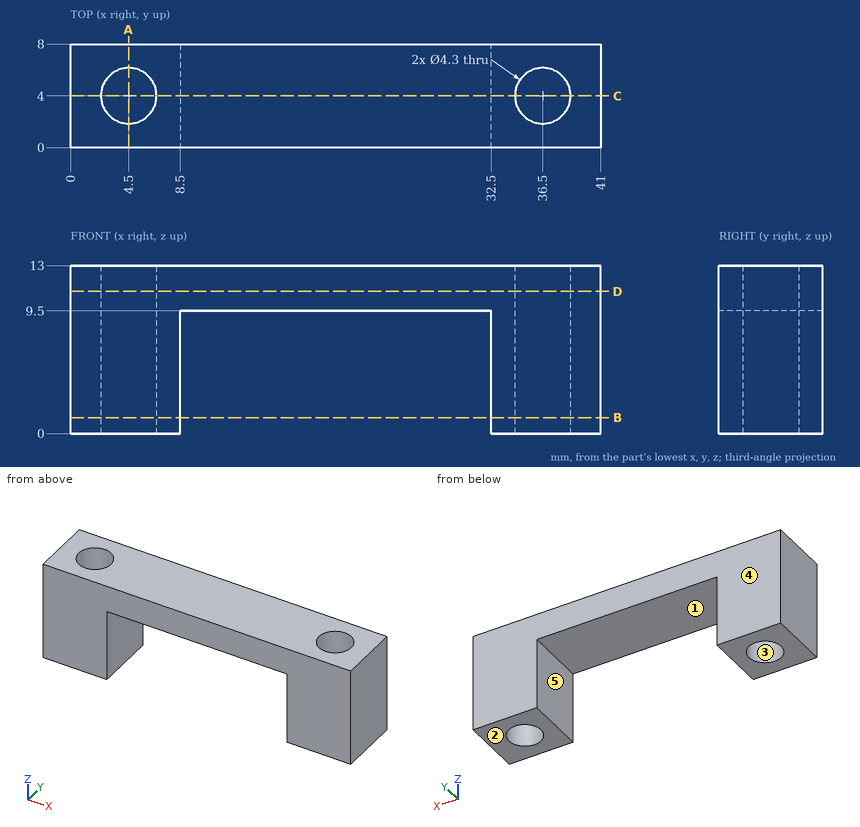
Drawing for the job (mm, zero at the part's lowest x, y, z). A direction names the side the tool comes from. Round coordinates to 2 decimals unless told otherwise and drop trailing zeros. Write each loop counter-clockwise with the first axis right and the second up, starting at its lowest first coordinate (ties: lowest second). Pieces come first, ordered by that corner, then holes. Notation, with made-up numbers: (4, -35.5) - (52, -35.5) arc R21 cw to (52, -1.5) - close; hole circle Ø11 at (24, 25). An arc over 180 degrees is marked (long way). Return JSON: item names as keys, results as strings. Group by question number.
Item 1: Band-saw the part on A-A on x = 4.5. List the corners of the cut face in (y, z), plus the area to 3 significant figures.
Item 2: Mould opens along Y. For the marked faces 3, 4 and 5 say: +Y half, -Y half, draft (parallel to the pull), parting line (faces both ways), or undercut.
Item 3: Flat gauge pins, fed straight in: pin 1 Ø1 at (x, y) = (26.5, 7) entering from -Z; pin 2 Ø2.5 at (x, y) = (36.5, 4) entering from +Z; pin 3 Ø2 at (y, z) = (5.5, 5.5) entering from -X. Where does each tip first touch, or does it go through?
Item 4: 3-axis set-ups, long thin cutter, end or side, ignore diameter. For the marked faces 1 and 2: which of +Z, -Z, +X, -X, +Y, -Y reach the whole face in a straight line?
Item 5: Band-saw the part on B-B on z = 1.25. List the corners of the cut face in (x, y).
Item 6: Band-saw the part on C-C on y = 4. List the corners of the cut face in (x, z).
Item 7: Probe probe 1 along Y at (x, z) = (4.5, 5.5); probe 2 along X at (y, z) = (1.75, 6.75); probe 3 along X at (y, z) = (4.5, 9.75). List the from-to ranges inside material, lowest first.
Item 8: Band-saw the part on D-D on z = 11. List the corners of the cut face in (x, y), plus the area to 3 significant figures.
Resolved:
{
 "1": {"outline": "(0, 0) - (1.85, 0) - (1.85, 13) - (0, 13) - close; (6.15, 0) - (8, 0) - (8, 13) - (6.15, 13) - close", "area": "48.1 mm²"},
 "2": {"face 3": "undercut", "face 4": "+Y half", "face 5": "draft"},
 "3": {"pin 1": "stops at z = 9.5", "pin 2": "passes through", "pin 3": "stops at x = 0"},
 "4": {"face 1": "-Z, +Y, -Y", "face 2": "-Z, +X, -X, +Y, -Y"},
 "5": {"outline": "(0, 0) - (8.5, 0) - (8.5, 8) - (0, 8) - close; (32.5, 0) - (41, 0) - (41, 8) - (32.5, 8) - close; hole circle Ø4.3 at (4.5, 4); hole circle Ø4.3 at (36.5, 4)"},
 "6": {"outline": "(0, 0) - (2.35, 0) - (2.35, 13) - (0, 13) - close; (6.65, 0) - (8.5, 0) - (8.5, 9.5) - (32.5, 9.5) - (32.5, 0) - (34.35, 0) - (34.35, 13) - (6.65, 13) - close; (38.65, 0) - (41, 0) - (41, 13) - (38.65, 13) - close"},
 "7": {"probe 1": "y = 0 to 1.85, 6.15 to 8", "probe 2": "x = 0 to 8.5, 32.5 to 41", "probe 3": "x = 0 to 2.41, 6.59 to 34.41, 38.59 to 41"},
 "8": {"outline": "(0, 0) - (41, 0) - (41, 8) - (0, 8) - close; hole circle Ø4.3 at (4.5, 4); hole circle Ø4.3 at (36.5, 4)", "area": "299 mm²"}
}
